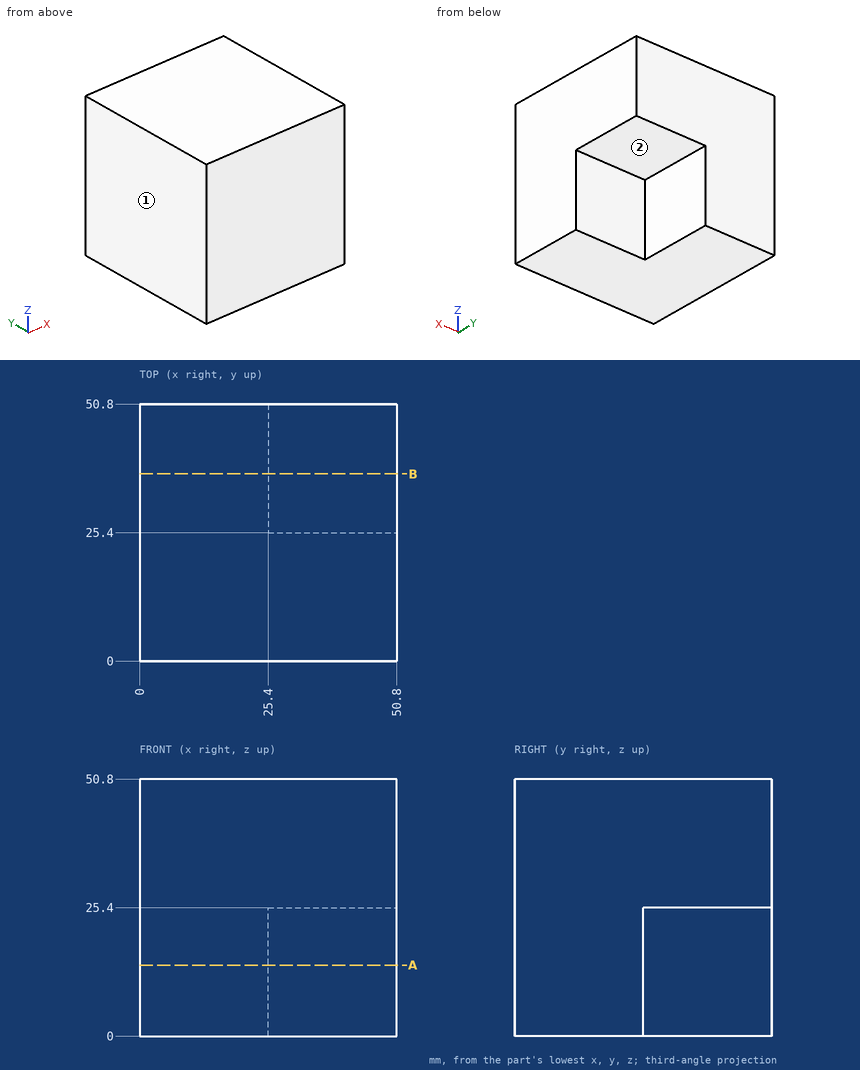
Drawing for the job (mm, zero at the part's lowest x, y, z). A direction names the side the tool comes from. Round coordinates to 2 decimals unless told otherwise and drop trailing zeros. Write each loop counter-clockwise with the first axis right and the second up, starting at its lowest first coordinate (ties: lowest second). Pieces come first, ordered by that corner, then holes. Notation, with made-up numbers: M -31.75,17.25 L -4.75,17.25 A29 cw -4.75,39.25 Z; hole C 65,3.5 d9. An arc over 180 degrees is marked long. Answer as a JSON object with one key per item and string values. Group by question number.
(1) Which spindle directions (+Z, -Z, +X, -X, +Y, -Y) get a long thin tool onto all of the face, cutting with end or side? Do the marked faces 1 and 2. Say none if no direction does.
(2) Flat gauge pin, fed straight in: pin 1 (10 mm diameter, centred on x = 39.5, y = 42.5, fed in from -Z). Where does the tip first touch, or does it go through?
(3) Drill centre lines: L1, parallel to Z at x = 41, y = 48.5; L2, parallel to Y at x = 47, z = 22.5. Where is each one in solid material? Low to high.
(4) Cut at B-B (y = 37). Give the cut face in (x, z), and give its area (3 significant figures).
(5) Cut at A-A (z = 14). Give the cut face in (x, y).
Responses:
{
 "1": {"face 1": "+Z, -Z, -X, +Y, -Y", "face 2": "-Z, +X, +Y"},
 "2": {"pin 1": "stops at z = 25.4"},
 "3": {"L1": "z = 25.4 to 50.8", "L2": "y = 0 to 25.4"},
 "4": {"outline": "M 0,0 L 25.4,0 L 25.4,25.4 L 50.8,25.4 L 50.8,50.8 L 0,50.8 Z", "area": "1,940 mm2"},
 "5": {"outline": "M 0,0 L 50.8,0 L 50.8,25.4 L 25.4,25.4 L 25.4,50.8 L 0,50.8 Z"}
}
